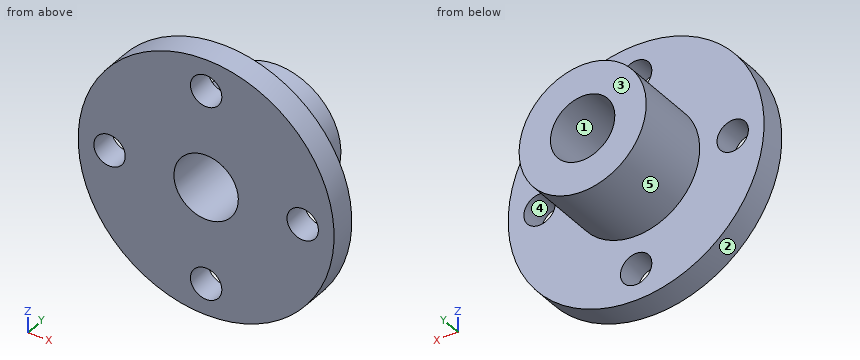
```python
from build123d import *

# Parameters (mm, degrees)
SKETCH1_R           = 15.9
SKETCH1_R_2         = 4
BOSS_EXTRUDE1_DEPTH = 13.05
CUT_EXTRUDE1_START  = -9.8
SKETCH2_R           = 15.9
SKETCH2_R_2         = 7.9
CUT_EXTRUDE1_DEPTH  = 9.8
SKETCH3_R           = 1.95
CUT_EXTRUDE2_DEPTH  = 9.8


with BuildPart() as part:
    # Sketch1 → Boss-Extrude1 (new body)
    with BuildSketch(Plane(origin=(0, 0, 0), x_dir=(1, 0, 0), z_dir=(0, 1, 0))):
        with Locations(Location((0, 0, 0), (0, 0, 270))):
            Circle(SKETCH1_R)
        with Locations(Location((0, 0, 0), (0, 0, 270))):
            Circle(SKETCH1_R_2, mode=Mode.SUBTRACT)
    extrude(amount=BOSS_EXTRUDE1_DEPTH)

    # Sketch2 → Cut-Extrude1 (cut)
    with BuildSketch(Plane(origin=(0, 13.05, 0), x_dir=(1, 0, 0), z_dir=(0, 1, 0)).offset(CUT_EXTRUDE1_START)):
        with Locations(Location((0, 0, 0), (0, 0, 270))):
            Circle(SKETCH2_R)
        with Locations(Location((0, 0, 0), (0, 0, 270))):
            Circle(SKETCH2_R_2, mode=Mode.SUBTRACT)
    extrude(amount=CUT_EXTRUDE1_DEPTH, mode=Mode.SUBTRACT)

    # Sketch3 → Cut-Extrude2 (cut)
    with BuildSketch(Plane(origin=(0, 3.25, 0), x_dir=(1, 0, 0), z_dir=(0, 1, 0))):
        with Locations(Location((0, 12, 0), (0, 0, 270))):
            Circle(SKETCH3_R)
        with Locations(Location((12, 0, 0), (0, 0, 270))):
            Circle(SKETCH3_R)
        with Locations(Location((0, -12, 0), (0, 0, 270))):
            Circle(SKETCH3_R)
        with Locations(Location((-12, 0, 0), (0, 0, 270))):
            Circle(SKETCH3_R)
    extrude(amount=-CUT_EXTRUDE2_DEPTH, mode=Mode.SUBTRACT)


solid = part.part
```
For this review, take the finished solid that the model builds, in its own axes (mm). Face numbers are marked on the shaded views. A direction names the side the tool comes from. Give positions to 0.01 mm unless a question says otherwise; leave off trailing zeros. Order: outer loops, then holes, each group sorted by start corner. A loop starts at its lowest first (then second) coordinate and runs counter-clockwise, first axis right, second up.
1) Take a section at B-B (z = -13). Give the boundary of the cut face in (x, y).
2) Take a section at A-A (x = 0). Give the boundary of the cut face in (y, z).
3) Take a section at D-D (y = 2.75). Give the boundary of the cut face in (x, z), then the cut area to 3 significant figures.
4) Insertion check: pin 1 (1.5 mm diameter, centred on y = 2.5, z = 7.5, fed in from +X); pin 2 (1 mm diameter, centred on x = -10.5, z = 3, fed in from +Y); pin 3 (6 mm diameter, centred on y = 10, z = -5, fed in from -X). Each pin has a flat end and moves straight along its axis. Give the tip position at first contact, or say it passes through.
5) Take a section at C-C (x = -11). Give the boundary of the cut face in (y, z), then the cut area to 3 significant figures.
6) Wall thickness on line 1 (X direction, y = 7.75, z = 0); line 2 (Y direction, x = -12, z = 5); line 3 (Z direction, x = 1, y = 9.75): over which ranges is each line inside the solid? List them lowest first.
7) For the marked faces 4 and 5, list the 3-axis set-ups (+Z, -Z, +X, -X, +Y, -Y) from which the entire face can be reached by the end or side of a thin tool; tool diameter is ignored.
8) The part is to be moulded in two halves that separate along X. For the marked faces 1, 2 and 3, say which applies: released by +X, released by -X, zero draft, split by the parting line, or undercut.
Derived:
1. outline: (-9.15, 0) - (-1.67, 0) - (-1.67, 3.25) - (-9.15, 3.25) - close; (1.67, 0) - (9.15, 0) - (9.15, 3.25) - (1.67, 3.25) - close
2. outline: (0, -15.9) - (3.25, -15.9) - (3.25, -13.95) - (0, -13.95) - close; (0, -10.05) - (3.25, -10.05) - (3.25, -7.9) - (13.05, -7.9) - (13.05, -4) - (0, -4) - close; (0, 4) - (13.05, 4) - (13.05, 7.9) - (3.25, 7.9) - (3.25, 10.05) - (0, 10.05) - close; (0, 13.95) - (3.25, 13.95) - (3.25, 15.9) - (0, 15.9) - close
3. outline: circle Ø31.8 at (0, 0); hole circle Ø3.9 at (-12, 0); hole circle Ø8 at (0, 0); hole circle Ø3.9 at (0, -12); hole circle Ø3.9 at (0, 12); hole circle Ø3.9 at (12, 0)
3. area: 696 mm2
4. pin 1: stops at x = 14.4
4. pin 2: stops at y = 3.25
4. pin 3: stops at x = -7.64
5. outline: (0, -11.48) - (3.25, -11.48) - (3.25, -1.67) - (0, -1.67) - close; (0, 1.67) - (3.25, 1.67) - (3.25, 11.48) - (0, 11.48) - close
5. area: 63.7 mm2
6. line 1: x = -7.9 to -4, 4 to 7.9
6. line 2: y = 0 to 3.25
6. line 3: z = -7.84 to -3.87, 3.87 to 7.84
7. face 4: +Y, -Y
7. face 5: +Y
8. face 1: undercut
8. face 2: split by the parting line
8. face 3: zero draft
